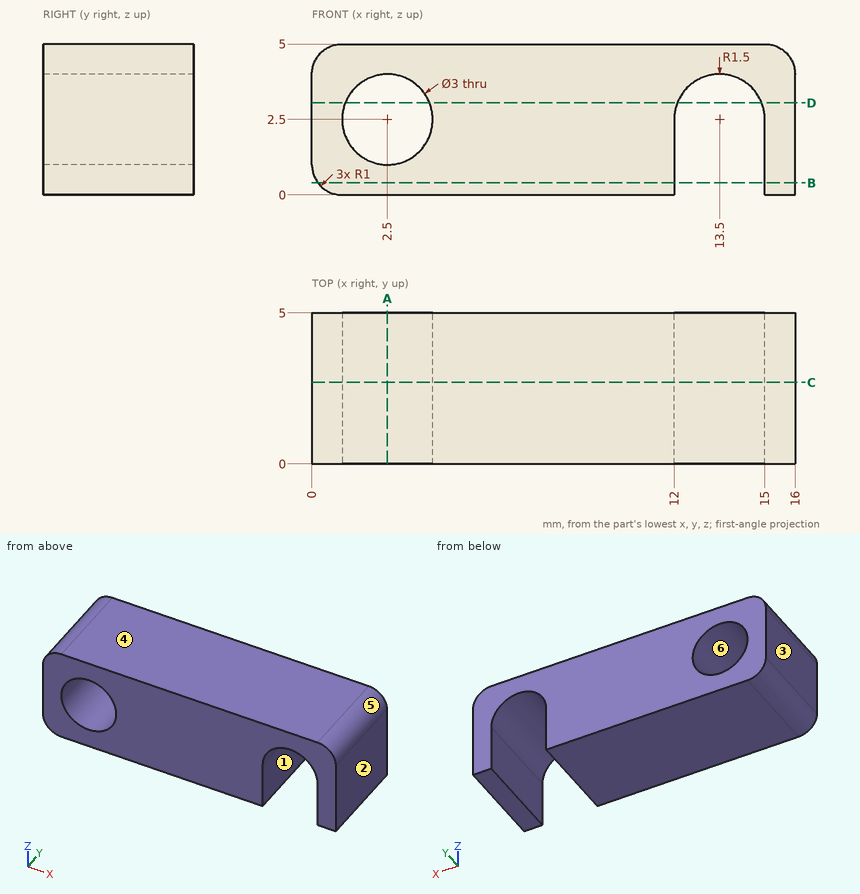
Geometry: see drawing. Coordinates: mm, zero at the bounding-box minimum. A direction names the side the tool comes from. Give positions to 0.01 mm unless a question says otherwise; leave off trailing zeros. Order: outer loops, then holes, each group sorted by start corner. A loop starts at its lowest first (then second) coordinate and runs counter-clockwise, first axis right, second up. Notation, with made-up numbers: (-36, 13) -> (10, 13) arc R16 cw to (10, 32) -> close; hole circle Ø7 at (16, 40). An arc over 180 degrees is marked (long way). Write each question's results on one line, items separated by ' | '.
1) Cut plane B-B (z = 0.4). Output: boundary loops of the cut face in (x, y).
Geometry says:
outline: (0.2, 0) -> (12, 0) -> (12, 5) -> (0.2, 5) -> close; (15, 0) -> (16, 0) -> (16, 5) -> (15, 5) -> close
2) Line query: line 1 along X through (y, z) = (0.8, 1.5); line 2 along Z through (x, y) = (2.5, 4.05); line 3 along X through (y, z) = (0.65, 2). Output: solid intervals per line, ascending.
Geometry says:
line 1: x = 0 to 1.38, 3.62 to 12, 15 to 16 | line 2: z = 0 to 1, 4 to 5 | line 3: x = 0 to 1.09, 3.91 to 12, 15 to 16
3) Cut plane C-C (y = 2.7). Output: boundary loops of the cut face in (x, z), and give its area (3 significant figures).
Geometry says:
outline: (0, 1) arc R1 ccw to (1, 0) -> (12, 0) -> (12, 2.5) arc R1.5 cw to (15, 2.5) -> (15, 0) -> (16, 0) -> (16, 4) arc R1 ccw to (15, 5) -> (1, 5) arc R1 ccw to (0, 4) -> close; hole circle Ø3 at (2.5, 2.5) | area: 61.3 mm²
4) Set-up query: the marked faces 1 and 2. Return all of +Z, -Z, +X, -X, +Y, -Y with unobstructed straight access to the full face (end or side cutting, diameter ignored); none if empty.
Geometry says:
face 1: -Z, +Y, -Y | face 2: +Z, -Z, +X, +Y, -Y
5) First-contact query: pin 1 Ø1.5 at (y, z) = (1, 3.5) entering from -X. Flat tip, straight axial feed; report the tip coordinate or a pass-through.
Geometry says:
pin 1: stops at x = 0
6) Draft query along X for the marked faces 3, 4, 5 and 6. Return one class per face: released by +X, released by -X, zero draft, split by the parting line, or undercut.
Geometry says:
face 3: released by -X | face 4: zero draft | face 5: released by +X | face 6: undercut
7) Cut plane A-A (x = 2.5). Output: boundary loops of the cut face in (y, z), and give its area (3 significant figures).
Geometry says:
outline: (0, 0) -> (5, 0) -> (5, 1) -> (0, 1) -> close; (0, 4) -> (5, 4) -> (5, 5) -> (0, 5) -> close | area: 10.0 mm²
8) Cut plane D-D (z = 3.05). Output: boundary loops of the cut face in (x, y).
Geometry says:
outline: (0, 0) -> (1.1, 0) -> (1.1, 5) -> (0, 5) -> close; (3.9, 0) -> (12.1, 0) -> (12.1, 5) -> (3.9, 5) -> close; (14.9, 0) -> (16, 0) -> (16, 5) -> (14.9, 5) -> close
